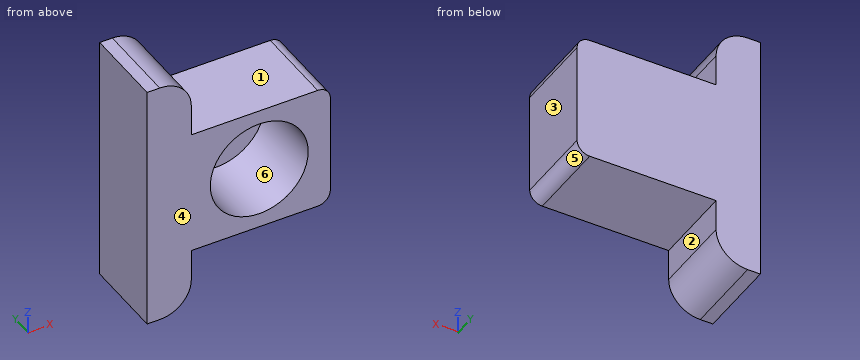
from build123d import *

# Parameters (mm, degrees)
F0_W     = 29
F0_H     = 13
F1_DEPTH = 20
F2_R     = 7.75
F3_DEPTH = 12
F5_DEPTH = 10
F6_W     = 7
F6_H     = 13
F7_DEPTH = 10
F8_R     = 5
F9_R     = 2


with BuildPart() as f1:
    # F0 (on Top) → F1 (new body)
    with BuildSketch(Plane.XY):
        with Locations((14.5, 6.5)):
            Rectangle(F0_W, F0_H)
    extrude(amount=F1_DEPTH)

    # F2 (on face) → F3 (cut)
    with BuildSketch(Plane.XZ):
        with Locations((17.75, 10)):
            Circle(F2_R)
    extrude(amount=-F3_DEPTH, mode=Mode.SUBTRACT)

    # F4 (on face) → F5 (join)
    with BuildSketch(Plane.XY.offset(20)):
        Polygon((2, 0), (7, 0), (7, 13), (0, 13), (0, 0), align=None)
    extrude(amount=F5_DEPTH)

    # F6 (on face) → F7 (join)
    with BuildSketch(Plane(origin=(0, 0, 0), x_dir=(1, 0, 0), z_dir=(0, 0, -1))):
        with Locations((3.5, -6.5)):
            Rectangle(F6_W, F6_H)
    extrude(amount=F7_DEPTH)

    # F8
    f8_edges = [f1.edges().sort_by_distance(p)[0] for p in [
        (7, 6.5, 30),
        (7, 6.5, -10),
    ]]
    fillet(f8_edges, radius=F8_R)

    # F9
    f9_edges = [f1.edges().sort_by_distance(p)[0] for p in [
        (29, 6.5, 20),
        (29, 6.5, 0),
    ]]
    fillet(f9_edges, radius=F9_R)


solid = f1.part
Build history of the part. All positions in model axes, mm. Face numbers are marked on the shaded views. A direction names the side the tool comes from. Round coordinates to 2 decimals unless told otherwise and drop trailing zeros. Write each loop counter-clockwise with the first axis right and the second up, starting at its lowest first coordinate (ties: lowest second). Pieces come first, ordered by that corner, then holes. Notation, with made-up numbers: M 16.5,84 L 70.5,84 A11 ccw 70.5,101 Z; hole C -3,-14 d3. An arc over 180 degrees is marked long. Answer in a Markdown table with one row per item.
1. Saw through at A-A (y = 8.5). List the corners of the cut face in (x, z), and give its area (3 significant figures).
Geometry check:
| item | result |
|---|---|
| outline | M 0,-10 L 2,-10 A5 ccw 7,-5 L 7,0 L 27,0 A2 ccw 29,2 L 29,18 A2 ccw 27,20 L 7,20 L 7,25 A5 ccw 2,30 L 0,30 Z; hole C 17.75,10 d15.5 |
| area | 519 mm2 |
2. Probe L1, parallel to Z at x = 17.75, y = 5.5; L2, parallel to Y at x = 23.5, z = 10.5; L3, parallel to Z at x = 27, y = 7. List the from-to ranges inside material, lowest first. Write a range as [from, to].
Geometry check:
| item | result |
|---|---|
| L1 | [0, 2.25], [17.75, 20] |
| L2 | [12, 13] |
| L3 | [0, 20] |
3. Which spindle directions (+Z, -Z, +X, -X, +Y, -Y) get a long thin tool onto all of the face, cutting with end or side? Do the marked faces 1, 2 and 3. Say none if no direction does.
Geometry check:
| item | result |
|---|---|
| face 1 | +Z, +X, +Y, -Y |
| face 2 | -Z, +X, +Y, -Y |
| face 3 | +Z, -Z, +X, +Y, -Y |
4. Saw through at D-D (z = -1.5). List the corners of the cut face in (x, y).
Geometry check:
| item | result |
|---|---|
| outline | M 0,0 L 7,0 L 7,13 L 0,13 Z |
5. Saw through at B-B (z = 10). List the corners of the cut face in (x, y), and give its area (3 significant figures).
Geometry check:
| item | result |
|---|---|
| outline | M 0,0 L 10,0 L 10,12 L 25.5,12 L 25.5,0 L 29,0 L 29,13 L 0,13 Z |
| area | 191 mm2 |
6. Flat gauge pins, fed straight in: P1, Ø4, axis at x = 20.5, z = 18, coming from the -Y side; P2, Ø6, axis at x = 13.5, y = 9.5, coming from the +Z side; P3, Ø4, axis at y = 8.5, z = -2.5, coming from the +X side; P4, Ø9.5, axis at x = 17.75, z = 10, coming from the -Y side. Where does each tip first touch, or does it go through?
Geometry check:
| item | result |
|---|---|
| P1 | y = 0 |
| P2 | z = 20 |
| P3 | x = 7 |
| P4 | y = 12 |
7. Saw through at C-C (x = 17.75). List the corners of the cut face in (y, z), and give its area (3 significant figures).
Geometry check:
| item | result |
|---|---|
| outline | M 0,0 L 13,0 L 13,20 L 0,20 L 0,17.75 L 12,17.75 L 12,2.25 L 0,2.25 Z |
| area | 74.0 mm2 |
8. Mould opens along X. For the marked faces 4, 5 and 6 say: +X half, -X half, draft (parallel to the pull), parting line (faces both ways), or undercut.
Geometry check:
| item | result |
|---|---|
| face 4 | draft |
| face 5 | +X half |
| face 6 | undercut |
